Input: dimensioned drawing with shaded views. Units: mm. Origin: part minimum x, y, z. A direction names the side the tool comes from. Coordinates: 2 decimals unless noted, no trailing zeros. Loops run counter-clockwise (first coordinate to the right, second up) from the corner with the lowest first, then second, coordinate; pieces in that order, holes last. Notation, with made-up numbers: M -7.5,81 L 34.5,81 A24 cw 34.5,106 Z; hole C -27.5,55.25 d4. An arc over 180 degrees is marked long. Write item = value, one per line. Start each with the question number.
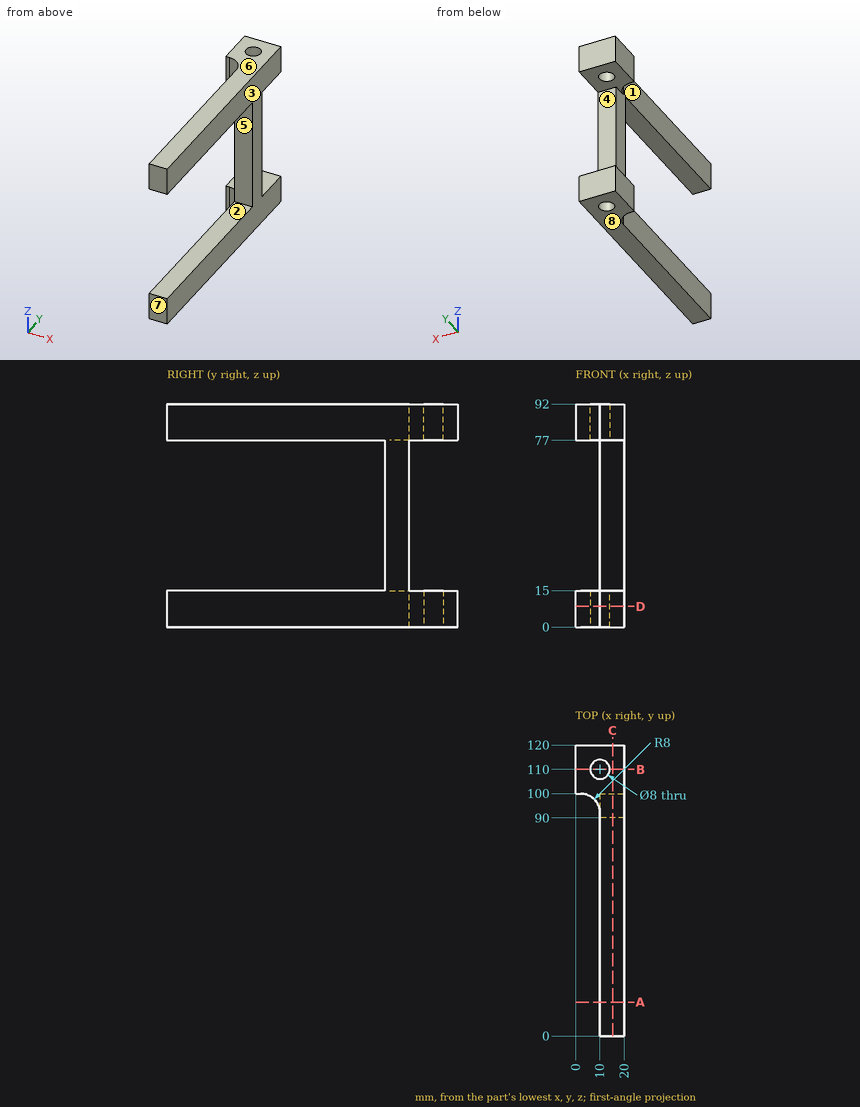
Item 1: Line query: line 1 (Z direction, x = 6, y = 114.5); line 2 (X direction, y = 59.5, z = 77.5); line 3 (Y direction, x = 11, z = 86). Output: solid intervals per line, ascending. Write a range as from..to.
Item 2: Section query D-D (z = 8.5). Return the cut outline in (x, y).
Item 3: First-contact query: pin 1 (1 mm diameter, centred on x = 9, z = 74, fed in from -Y); pin 2 (10.5 mm diameter, centred on x = 10, y = 110, fed in from +Z); pin 3 (1 mm diameter, centred on x = 1, z = 7.5, fed in from -Y); pin 4 (5 mm diameter, centred on y = 65.5, z = 12.5, fed in from -X). Flat tips, straight axial feed; report the tip coordinate or a pass-through.
Item 4: Reachability of the marked faces 1, 2, 3 and 4 from +Z, -Z, +X, -X, +Y, -Y: full face, straight path, thin tool, end or side. Return the list, or none.
Item 5: Section query B-B (y = 110). Return the cut outline in (x, z), plus the area to 3 significant figures.
Item 6: Pull-direction query (Z, two-part tool) for the marked faces 5, 6, 7 and 8; classes: released by +Z, released by -Z, zero draft, split by the parting line, or undercut.
Item 7: Section query A-A (y = 14). Return the cut outline in (x, z).
Item 8: Section query C-C (x = 15.25). Return the cut outline in (y, z), plus the area to 3 significant figures.
Verdict:
q1.line_1 = 0..15, 77..92
q1.line_2 = 10..20
q1.line_3 = 0..106.13, 113.87..120
q2.outline = M 0,100 L 2,100 A8 cw 10,92 L 10,0 L 20,0 L 20,120 L 0,120 Z; hole C 10,110 d8
q3.pin_1 = through
q3.pin_2 = 92
q3.pin_3 = 100
q3.pin_4 = 10
q4.face_1 = -X, -Y
q4.face_2 = +X, -X, -Y
q4.face_3 = +Z, -Z, +X, +Y, -Y
q4.face_4 = +X, -X, +Y
q5.outline = M 0,0 L 6,0 L 6,15 L 0,15 Z; M 0,77 L 6,77 L 6,92 L 0,92 Z; M 14,0 L 20,0 L 20,15 L 14,15 Z; M 14,77 L 20,77 L 20,92 L 14,92 Z
q5.area = 360 mm2
q6.face_5 = undercut
q6.face_6 = released by +Z
q6.face_7 = zero draft
q6.face_8 = released by -Z
q7.outline = M 10,0 L 20,0 L 20,15 L 10,15 Z; M 10,77 L 20,77 L 20,92 L 10,92 Z
q8.outline = M 0,0 L 120,0 L 120,15 L 100,15 L 100,77 L 120,77 L 120,92 L 0,92 L 0,77 L 90,77 L 90,15 L 0,15 Z
q8.area = 4,220 mm2
